For this review, take the finished solid that the model builds, in its own axes (mm). A direction names the side the tool comes from. Coordinates: 2 decimals unless noted, no trailing zeros. Write each loop counter-clockwise with the first axis right and the second up, starting at its lowest first coordinate (ties: lowest second). Pieces come first, ordered by that corner, then holes. Notation, with made-up numbers: (19, 84) - (64, 84) arc R29 cw to (64, 122) - close; hole circle Ø1 at (33, 59.5). An arc over 180 degrees is marked (long way). Use one line per item in the form item = value. Start each with the question number.
1) For L1, parallel to Y at x = -10, z = 0.45; L2, parallel to Y at x = 0, z = 8.75; L3, parallel to Z at x = -11.75, y = 8, list the stretches that pass through material, from the lowest coordinate up. Write a range as from..to.
2) We need section A-A (z = -2.5). Give the boundary of the cut face in (x, y).
3) We need section B-B (y = -9.25). Give the boundary of the cut face in (x, z), plus the area to 3 significant figures.
4) We need section D-D (z = 4.25). Give the boundary of the cut face in (x, y).
5) We need section C-C (x = -10). Give the boundary of the cut face in (y, z), plus the area to 3 significant figures.
6) Insertion check: P1, Ø1, axis at x = -10.5, z = -4.5, coming from the -Y side; P2, Ø1, axis at x = 6.5, y = 4, coming from the -Z side; P3, Ø1, axis at x = 10, z = -6, coming from the +Y side; P4, Ø2.5, axis at x = -10, y = -9.25, coming from the -Z side. Each pin has a flat end and moves straight along its axis. Give the tip position at first contact, or say it passes through.
7) Mouldability with a two-part tool opening along Y and no side actions: class faces 4 (the flat face through (10, 0, -10)), 5 (the cylindrical face through (-11.19, -10.16, 0.77)), 6 (the flat face through (10, 5, -5)) as pulls with the +Y half, pulls with the -Y half, needs draft (parallel to the pull), parting line crosses it, or undercut.
8) Tool access review of faces 1 (the flat face through (-8, 0, 5)), 2 (the flat face through (0, 8, 5)), 3 (the flat face through (8, 0, 5)): name each direction out of +Z, -Z, +X, -X, +Y, -Y from which nothing blocks a thin tool from reaching the whole face with its end or side.
```python
from build123d import *

# Parameters (mm, degrees)
SKETCH_1_W          = 26.5
SKETCH_1_H          = 24.5
SKETCH_1_R          = 1.5
EXTRUDE_1_DEPTH     = 1.57
SKETCH_3_W          = 16
SKETCH_3_H          = 16
EXTRUDE_2_DEPTH     = 7
SKETCH_4_R          = 8
EXTRUDE_3_DEPTH     = 4
SKETCH_5_R          = 5.8
CUT_EXTRUDE_1_DEPTH = 11
FILLET_1_R          = 2
SKETCH_6_W          = 2
SKETCH_6_H          = 10
EXTRUDE_4_DEPTH     = 10


with BuildPart() as part:
    # 草图1 → 凸台-拉伸1 (new body)
    with BuildSketch(Plane.XY):
        Rectangle(SKETCH_1_W, SKETCH_1_H)
        with Locations((-10, 9.25)):
            Circle(SKETCH_1_R, mode=Mode.SUBTRACT)
        with Locations((10, 9.25)):
            Circle(SKETCH_1_R, mode=Mode.SUBTRACT)
        with Locations((10, -9.25)):
            Circle(SKETCH_1_R, mode=Mode.SUBTRACT)
        with Locations((-10, -9.25)):
            Circle(SKETCH_1_R, mode=Mode.SUBTRACT)
    extrude(amount=EXTRUDE_1_DEPTH)

    # 草图3 → 凸台-拉伸2 (add)
    with BuildSketch(Plane.XY.offset(1.57)):
        Rectangle(SKETCH_3_W, SKETCH_3_H)
    extrude(amount=EXTRUDE_2_DEPTH)

    # 草图4 → 凸台-拉伸3 (add)
    with BuildSketch(Plane.XY.offset(8.57)):
        Circle(SKETCH_4_R)
    extrude(amount=EXTRUDE_3_DEPTH)

    # 草图5 → 切除-拉伸1 (cut)
    with BuildSketch(Plane.XY.offset(12.57)):
        Circle(SKETCH_5_R)
    extrude(amount=-CUT_EXTRUDE_1_DEPTH, mode=Mode.SUBTRACT)

    # 圆角1
    fillet_1_edges = [part.edges().sort_by_distance(p)[0] for p in [
        (13.25, -12.25, 0.785),
        (-13.25, -12.25, 0.785),
        (-13.25, 12.25, 0.785),
        (13.25, 12.25, 0.785),
    ]]
    fillet(fillet_1_edges, radius=FILLET_1_R)

    # 草图6 → 凸台-拉伸4 (add)
    with BuildSketch(Plane(origin=(0, 0, 0), x_dir=(-1, 0, 0), z_dir=(0, 0, -1))):
        with Locations((-10, 0)):
            Rectangle(SKETCH_6_W, SKETCH_6_H)
        with Locations((10, 0)):
            Rectangle(SKETCH_6_W, SKETCH_6_H)
    extrude(amount=EXTRUDE_4_DEPTH)


solid = part.part
```
Determined:
q1.L1 = -12.25..-10.75, -7.75..7.75, 10.75..12.25
q1.L2 = -8..-5.8, 5.8..8
q1.L3 = 0..1.57
q2.outline = (-11, -5) - (-9, -5) - (-9, 5) - (-11, 5) - close; (9, -5) - (11, -5) - (11, 5) - (9, 5) - close
q3.outline = (-13.25, 0) - (-11.5, 0) - (-11.5, 1.57) - (-13.25, 1.57) - close; (-8.5, 0) - (8.5, 0) - (8.5, 1.57) - (-8.5, 1.57) - close; (11.5, 0) - (13.25, 0) - (13.25, 1.57) - (11.5, 1.57) - close
q3.area = 32.2 mm²
q4.outline = (-8, -8) - (8, -8) - (8, 8) - (-8, 8) - close; hole circle Ø11.6 at (0, 0)
q5.outline = (-12.25, 0) - (-10.75, 0) - (-10.75, 1.57) - (-12.25, 1.57) - close; (-7.75, 0) - (-5, 0) - (-5, -10) - (5, -10) - (5, 0) - (7.75, 0) - (7.75, 1.57) - (-7.75, 1.57) - close; (10.75, 0) - (12.25, 0) - (12.25, 1.57) - (10.75, 1.57) - close
q5.area = 129 mm²
q6.P1 = -5
q6.P2 = 0
q6.P3 = 5
q6.P4 = through
q7.face_4 = needs draft
q7.face_5 = undercut
q7.face_6 = pulls with the +Y half
q8.face_1 = +Z, -X, +Y, -Y
q8.face_2 = +Z, +X, -X, +Y
q8.face_3 = +Z, +X, +Y, -Y
